Source: CAD feature listing. Evaluate the final solid. Frame: model axes, mm. Give positions to 0.01 mm unless a question says otherwise; leave off trailing zeros. Order: outer loops, then holes, each group sorted by start corner. A loop starts at its lowest first (then second) coordinate and runs counter-clockwise, first axis right, second up. Notation, with made-up numbers: M -21,-8 L 31,-8 A21 cw 31,8 Z; hole C 8,-13 d8. An arc over 180 degrees is marked long. Answer in a Markdown table with one row per item. Add a question column.
(1) Material intervals for line 1 along Y through (x, z) = (-136, -97.5), sorted ascending.
(2) Section query B-B, the plane x = 50. Return loops of the section in (y, z).
(3) Pin query (flat end, axial travel): P1, Ø2, axis at x = 106.5, z = -95.5, coming from the +Y side; P2, Ø3, axis at x = 175, y = 41.5, coming from the +Z side; P3, Ø2.5, axis at y = 68, z = -128, coming from the -X side. Return the tip coordinate at first contact, or that it passes through.
(4) Section query A-A, the plane z = -51. Return loops of the section in (x, y).
from build123d import *

# Parameters (mm, degrees)
ESQUISSE1_W        = 360
ESQUISSE1_H        = 260
BOSS_EXTRU_1_DEPTH = 5
ESQUISSE3_W        = 10
ESQUISSE3_H        = 5
BOSS_EXTRU_3_DEPTH = 100


with BuildPart() as part:
    # Esquisse1 → Boss.-Extru.1 (new body)
    with BuildSketch(Plane(origin=(0, 0, 0), x_dir=(1, 0, 0), z_dir=(0, 1, 0))):
        Rectangle(ESQUISSE1_W, ESQUISSE1_H)
    extrude(amount=BOSS_EXTRU_1_DEPTH)

    # Esquisse3 → Boss.-Extru.3 (add)
    with BuildSketch(Plane(origin=(0, 5, 0), x_dir=(1, 0, 0), z_dir=(0, 1, 0))):
        with Locations((175, 127.5)):
            Rectangle(ESQUISSE3_W, ESQUISSE3_H)
    extrude(amount=BOSS_EXTRU_3_DEPTH)


solid = part.part
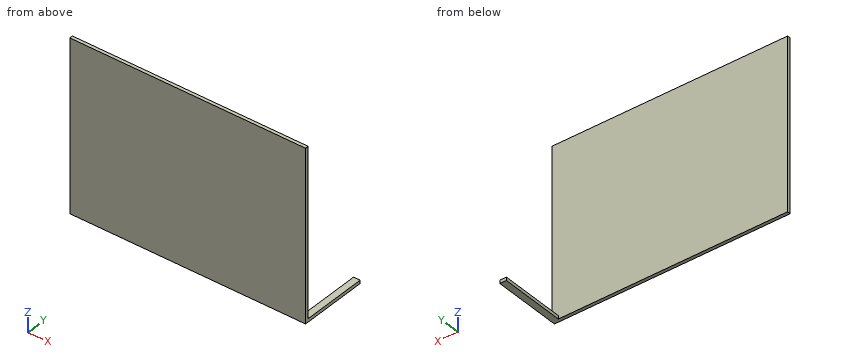
Values follow:
| question | item | result |
|---|---|---|
| 1 | line 1 | y = 0 to 5 |
| 2 | outline | M 0,-130 L 5,-130 L 5,130 L 0,130 Z |
| 3 | P1 | stops at y = 5 |
| 3 | P2 | stops at z = -125 |
| 3 | P3 | stops at x = 170 |
| 4 | outline | M -180,0 L 180,0 L 180,5 L -180,5 Z |
